from build123d import *

# Parameters (mm, degrees)
SKETCH1_R           = 9
SKETCH1_R_2         = 2.35
BOSS_EXTRUDE1_DEPTH = 3


with BuildPart() as part:
    # Sketch1 → Boss-Extrude1 (new body)
    with BuildSketch(Plane(origin=(0, 0, 0), x_dir=(1, 0, 0), z_dir=(0, 1, 0))):
        Circle(SKETCH1_R)
        with Locations((4.997281989, -0.164841493)):
            Circle(SKETCH1_R_2, mode=Mode.SUBTRACT)
        Polygon((-2.25, 0.9), (-2.25, -0.9), (-0.9, -0.9), (-0.9, -2.25), (0.9, -2.25), (0.9, -0.9), (2.25, -0.9), (2.25, 0.9), (0.9, 0.9), (0.9, 2.25), (-0.9, 2.25), (-0.9, 0.9), align=None, mode=Mode.SUBTRACT)
    extrude(amount=BOSS_EXTRUDE1_DEPTH)


solid = part.part
Design review of the part built by this model. Coordinates are the model's own, in mm. A direction names the side the tool comes from. Round coordinates to 2 decimals unless told otherwise and drop trailing zeros. Loops run counter-clockwise (first coordinate to the right, second up) from the corner with the lowest first, then second, coordinate; pieces in that order, holes last. Notation, with made-up numbers: M -19.5,73 L 37.5,73 A22 ccw 37.5,85 Z; hole C 73,-38 d2. An arc over 180 degrees is marked long. Answer as a JSON object with one key per item and string values.
Item 1: We need section B-B on y = 0.4. Give the boundary of the cut face in (x, z).
Answer sheet:
{"outline": "C 0,0 d18; hole M -2.25,-0.9 L -0.9,-0.9 L -0.9,-2.25 L 0.9,-2.25 L 0.9,-0.9 L 2.25,-0.9 L 2.25,0.9 L 0.9,0.9 L 0.9,2.25 L -0.9,2.25 L -0.9,0.9 L -2.25,0.9 Z; hole C 5,0.16 d4.7"}
Item 2: Machinability: for faces 1 (the flat face through (-2, 3, 2)), 2 (the flat face through (2.25, 1, 0)), which of the approach directions +Z, -Z, +X, -X, +Y, -Y give a long, thin tool a straight path to every point of the face, cutting with its end or side? Answer none if there is none.
Answer sheet:
{"face 1": "+Z, -Z, +X, -X, +Y", "face 2": "+Y, -Y"}
Item 3: We need section D-D on z = 5.75. Give the boundary of the cut face in (x, y), and give its area (3 significant figures).
Answer sheet:
{"outline": "M -6.92,0 L 6.92,0 L 6.92,3 L -6.92,3 Z", "area": "41.5 mm^2"}
Item 4: The part is to be moulded in two halves that separate along Z. For faces 3 (the flat face through (0, 1, -2.25)), 4 (the flat face through (0.9, 1, -2)), 5 (the flat face through (-2, 0, 2)), 6 (the cylindrical face through (-1.172, 1.479, -8.923)), say which applies: pulls with the +Z half, pulls with the -Z half, needs draft (parallel to the pull), parting line crosses it, or undercut.
Answer sheet:
{"face 3": "undercut", "face 4": "undercut", "face 5": "needs draft", "face 6": "parting line crosses it"}
Item 5: We need section A-A on x = 0. Give the boundary of the cut face in (y, z), and give its area (3 significant figures).
Answer sheet:
{"outline": "M 0,-9 L 3,-9 L 3,-2.25 L 0,-2.25 Z; M 0,2.25 L 3,2.25 L 3,9 L 0,9 Z", "area": "40.5 mm^2"}
Item 6: Clearance check with flat-ended pins moving along their axes: P1, Ø0.7, axis at x = 2, y = 1, coming from the -Z side; P2, Ø0.7, axis at y = 1, z = -1.5, coming from the -X side; P3, Ø1.1, axis at x = 2, y = 1.5, coming from the +Z side. State where each tip first meets the part, or that it passes through.
Answer sheet:
{"P1": "stops at z = -8.85", "P2": "stops at x = -8.93", "P3": "stops at z = 8.88"}
Item 7: We need section C-C on x = 5. Give the boundary of the cut face in (y, z).
Answer sheet:
{"outline": "M 0,-7.48 L 3,-7.48 L 3,-2.19 L 0,-2.19 Z; M 0,2.51 L 3,2.51 L 3,7.48 L 0,7.48 Z"}
Item 8: Wall thickness on L1, parallel to X at y = 2.3, z = 1; L2, parallel to X at y = 2.95, z = 0.25; L3, parallel to Z at x = 0, y = 0.3: over which ranges is each line inside the solid? List them lowest first. Write a range as from..to.
Answer sheet:
{"L1": "x = -8.94..-0.9, 0.9..2.8, 7.19..8.94", "L2": "x = -9..-2.25, 2.25..2.65, 7.35..9", "L3": "z = -9..-2.25, 2.25..9"}
